```python
from build123d import *

# Parameters (mm, degrees)
SKETCH1_W               = 66.294
SKETCH1_H               = 112.776
BOSS_EXTRUDE1_DEPTH     = 3.048
SKETCH2_W               = 66.294
SKETCH2_H               = 112.776
SKETCH2_W_2             = 60
SKETCH2_H_2             = 106.68
BOSS_EXTRUDE2_DEPTH     = 25.4
SKETCH3_W               = 12.7
SKETCH3_H               = 8.89
BOSS_EXTRUDE3_DEPTH     = 3.81
CUT_EXTRUDE1_REACH      = 93.563
SKETCH6_W               = 76.2
SKETCH6_H               = 7.62
SKETCH7_W               = 50.8
SKETCH7_H               = 42.7
BOSS_EXTRUDE4_DEPTH     = 6.35
CUT_EXTRUDE2_DEPTH      = 90.169551737
CUT_EXTRUDE2_DEPTH_BACK = 90.169551737
CUT_EXTRUDE3_START      = -6.35
SKETCH9_W               = 22.86
SKETCH9_H               = 9.7
CUT_EXTRUDE3_DEPTH      = 6.35
CUT_EXTRUDE4_REACH      = 76.089
SKETCH4_R               = 1.7
SKETCH4_R_2             = 1.72


with BuildPart() as part:
    # Sketch1 → Boss-Extrude1 (new body)
    with BuildSketch(Plane(origin=(0, 0, 0), x_dir=(1, 0, 0), z_dir=(0, 1, 0))):
        Rectangle(SKETCH1_W, SKETCH1_H)
    extrude(amount=BOSS_EXTRUDE1_DEPTH)

    # Sketch2 → Boss-Extrude2 (add)
    with BuildSketch(Plane(origin=(0, 3.048, 0), x_dir=(1, 0, 0), z_dir=(0, 1, 0))):
        Rectangle(SKETCH2_W, SKETCH2_H)
        Rectangle(SKETCH2_W_2, SKETCH2_H_2, mode=Mode.SUBTRACT)
    extrude(amount=BOSS_EXTRUDE2_DEPTH)

    # Sketch3 → Boss-Extrude3 (add)
    with BuildSketch(Plane(origin=(0, 28.448, 0), x_dir=(1, 0, 0), z_dir=(0, 1, 0))):
        with Locations((-23.65, 48.895)):
            Rectangle(SKETCH3_W, SKETCH3_H)
        with Locations((-23.65, -48.895)):
            Rectangle(SKETCH3_W, SKETCH3_H)
        with Locations((23.65, 48.895)):
            Rectangle(SKETCH3_W, SKETCH3_H)
        with Locations((23.65, -48.895)):
            Rectangle(SKETCH3_W, SKETCH3_H)
    extrude(amount=-BOSS_EXTRUDE3_DEPTH)

    # Sketch6 → Cut-Extrude1 (cut, up to next)
    with BuildSketch(Plane(origin=(33.147, 0, 0), x_dir=(0, 0, -1), z_dir=(1, 0, 0)), mode=Mode.PRIVATE) as cut_extrude1_sk1:
        with Locations((0, 6.858)):
            Rectangle(SKETCH6_W, SKETCH6_H)
    cut_extrude1_tool1 = extrude(cut_extrude1_sk1.sketch, amount=-CUT_EXTRUDE1_REACH, mode=Mode.PRIVATE) & part.part
    add(cut_extrude1_tool1.solids().sort_by_distance((33.147, 6.858, 0))[0], mode=Mode.SUBTRACT)

    # Sketch7 → Boss-Extrude4 (add)
    with BuildSketch(Plane.XZ):
        Rectangle(SKETCH7_W, SKETCH7_H)
    extrude(amount=BOSS_EXTRUDE4_DEPTH)

    # Sketch8 → Cut-Extrude2 (cut, two sides: drawn at the far end of the back side and taken through both)
    with BuildSketch(Plane.XY.offset(21.35).offset(-CUT_EXTRUDE2_DEPTH_BACK)):
        Polygon((-3.81, -3.175), (-3.81, 0), (-25.4, 0), (-25.4, -6.35), (-11.43, -6.35), (-11.43, -3.175), align=None)
        Polygon((25.4, 0), (3.81, 0), (3.81, -3.175), (11.43, -3.175), (11.43, -6.35), (25.4, -6.35), align=None)
    extrude(amount=CUT_EXTRUDE2_DEPTH + CUT_EXTRUDE2_DEPTH_BACK, mode=Mode.SUBTRACT)

    # Sketch9 → Cut-Extrude3 (cut)
    with BuildSketch(Plane.XZ.offset(6.35).offset(CUT_EXTRUDE3_START)):
        with Locations((0, 16.5)):
            Rectangle(SKETCH9_W, SKETCH9_H)
    extrude(amount=CUT_EXTRUDE3_DEPTH, mode=Mode.SUBTRACT)

    # Sketch4 → Cut-Extrude4 (cut, up to next)
    with BuildSketch(Plane(origin=(0, 28.448, 0), x_dir=(1, 0, 0), z_dir=(0, 1, 0)), mode=Mode.PRIVATE) as cut_extrude4_sk1:
        with Locations(Location((-23.65, 50.165, 0), (0, 0, 270))):
            Circle(SKETCH4_R)
    cut_extrude4_tool1 = extrude(cut_extrude4_sk1.sketch, amount=-CUT_EXTRUDE4_REACH, mode=Mode.PRIVATE) & part.part
    # Sketch4 → Cut-Extrude4 (cut, up to next)
    with BuildSketch(Plane(origin=(0, 28.448, 0), x_dir=(1, 0, 0), z_dir=(0, 1, 0)), mode=Mode.PRIVATE) as cut_extrude4_sk2:
        with Locations(Location((23.65, 50.165, 0), (0, 0, 270))):
            Circle(SKETCH4_R)
    cut_extrude4_tool2 = extrude(cut_extrude4_sk2.sketch, amount=-CUT_EXTRUDE4_REACH, mode=Mode.PRIVATE) & part.part
    # Sketch4 → Cut-Extrude4 (cut, up to next)
    with BuildSketch(Plane(origin=(0, 28.448, 0), x_dir=(1, 0, 0), z_dir=(0, 1, 0)), mode=Mode.PRIVATE) as cut_extrude4_sk3:
        with Locations(Location((23.65, -50.165, 0), (0, 0, 270))):
            Circle(SKETCH4_R_2)
    cut_extrude4_tool3 = extrude(cut_extrude4_sk3.sketch, amount=-CUT_EXTRUDE4_REACH, mode=Mode.PRIVATE) & part.part
    # Sketch4 → Cut-Extrude4 (cut, up to next)
    with BuildSketch(Plane(origin=(0, 28.448, 0), x_dir=(1, 0, 0), z_dir=(0, 1, 0)), mode=Mode.PRIVATE) as cut_extrude4_sk4:
        with Locations(Location((-23.65, -50.165, 0), (0, 0, 270))):
            Circle(SKETCH4_R)
    cut_extrude4_tool4 = extrude(cut_extrude4_sk4.sketch, amount=-CUT_EXTRUDE4_REACH, mode=Mode.PRIVATE) & part.part
    add(cut_extrude4_tool1.solids().sort_by_distance((-23.65, 28.448, -50.165))[0], mode=Mode.SUBTRACT)
    add(cut_extrude4_tool2.solids().sort_by_distance((23.65, 28.448, -50.165))[0], mode=Mode.SUBTRACT)
    add(cut_extrude4_tool3.solids().sort_by_distance((23.65, 28.448, 50.165))[0], mode=Mode.SUBTRACT)
    add(cut_extrude4_tool4.solids().sort_by_distance((-23.65, 28.448, 50.165))[0], mode=Mode.SUBTRACT)


solid = part.part
```
Part model, mm, in its own coordinate system. A direction names the side the tool comes from. Round coordinates to 2 decimals unless told otherwise and drop trailing zeros. Loops run counter-clockwise (first coordinate to the right, second up) from the corner with the lowest first, then second, coordinate; pieces in that order, holes last.
1. 3-axis set-ups, long thin cutter, end or side, ignore diameter. For faces 1 (the face through (0, -4, 11.65)), 2 (the face through (32, 7, 38.1)), 3 (the face through (-25.16, 26.57, 50.95)), 4 (the face through (-8, -3.175, -5)), 5 (the face through (-30, 16, 1)): which of +Z, -Z, +X, -X, +Y, -Y reach the whole face in a straight line?
Solutions:
face 1: +Z, +X, -X, -Y
face 2: +X
face 3: +Y
face 4: +Z, -Z, -X
face 5: none
2. Slice it at B-B (z = 24). Give the cut face in (x, y).
Solutions:
outline: (-33.15, 0) - (33.15, 0) - (33.15, 3.05) - (-30, 3.05) - (-30, 28.45) - (-33.15, 28.45) - close; (30, 10.67) - (33.15, 10.67) - (33.15, 28.45) - (30, 28.45) - close
3. Slice it at C-C (x = 23.65). Give the cut face in (y, z) (3 decimals), and give its area (3 significant figures).
Solutions:
outline: (0, -56.388) - (28.448, -56.388) - (28.448, -51.865) - (24.638, -51.865) - (24.638, -53.34) - (3.048, -53.34) - (3.048, 53.34) - (24.638, 53.34) - (24.638, 51.885) - (28.448, 51.885) - (28.448, 56.388) - (0, 56.388) - close; (24.638, -48.465) - (28.448, -48.465) - (28.448, -44.45) - (24.638, -44.45) - close; (24.638, 44.45) - (28.448, 44.45) - (28.448, 48.445) - (24.638, 48.445) - close
area: 540 mm2
4. Slice it at D-D (z = 6). Give the cut face in (x, y) (3 decimals), and give its area (3 significant figures).
Solutions:
outline: (-33.147, 0) - (-3.81, 0) - (-3.81, -3.175) - (-11.43, -3.175) - (-11.43, -6.35) - (11.43, -6.35) - (11.43, -3.175) - (3.81, -3.175) - (3.81, 0) - (33.147, 0) - (33.147, 3.048) - (-30, 3.048) - (-30, 28.448) - (-33.147, 28.448) - close; (30, 10.668) - (33.147, 10.668) - (33.147, 28.448) - (30, 28.448) - close
area: 435 mm2
5. Flat gauge pins, fed straight in: pin 1 (6 mm diameter, centred on x = 23.5, z = 26.5, fed in from +Y); pin 2 (4 mm diameter, centred on x = 23.65, z = 50.165, fed in from -Y); pin 3 (4 mm diameter, centred on x = -11.5, z = 7.5, fed in from -Y); pin 4 (1.6 mm diameter, centred on y = -4.5, z = 2.5, fed in from +X). Where does each tip first touch, or does it go through?
Solutions:
pin 1: stops at y = 3.05
pin 2: stops at y = 0
pin 3: stops at y = -6.35
pin 4: stops at x = 11.43
6. Slice it at A-A (x = -9). Give the cut face in (y, z) (3 decimals), and give its area (3 significant figures).
Solutions:
outline: (-6.35, -21.35) - (-3.175, -21.35) - (-3.175, 11.65) - (-6.35, 11.65) - close; (0, -56.388) - (28.448, -56.388) - (28.448, -53.34) - (3.048, -53.34) - (3.048, 53.34) - (28.448, 53.34) - (28.448, 56.388) - (0, 56.388) - close
area: 603 mm2
7. Drill centre lines: line 1 along X through (y, z) = (20.5, -24.5); line 2 along Z through (x, y) = (-5, 21); line 3 along Z through (x, y) = (-23, 27). Where is each one in solid material? Low to high.
Solutions:
line 1: x = -33.15 to -30, 30 to 33.15
line 2: z = -56.39 to -53.34, 53.34 to 56.39
line 3: z = -56.39 to -51.74, -48.59 to -44.45, 44.45 to 48.59, 51.74 to 56.39
8. Two-plate mould, pull along X, no slides. Class faces 6 (the face through (17.3, 27, 49)), 7 (the face through (-33.147, 14, 1)), 8 (the face through (32, 10.668, 1)), 9 (the face through (-17.3, 27, 49)): pulls with the +X half, pulls with the -X half, needs draft (parallel to the pull), parting line crosses it, or undercut.
Solutions:
face 6: undercut
face 7: pulls with the -X half
face 8: needs draft
face 9: undercut
